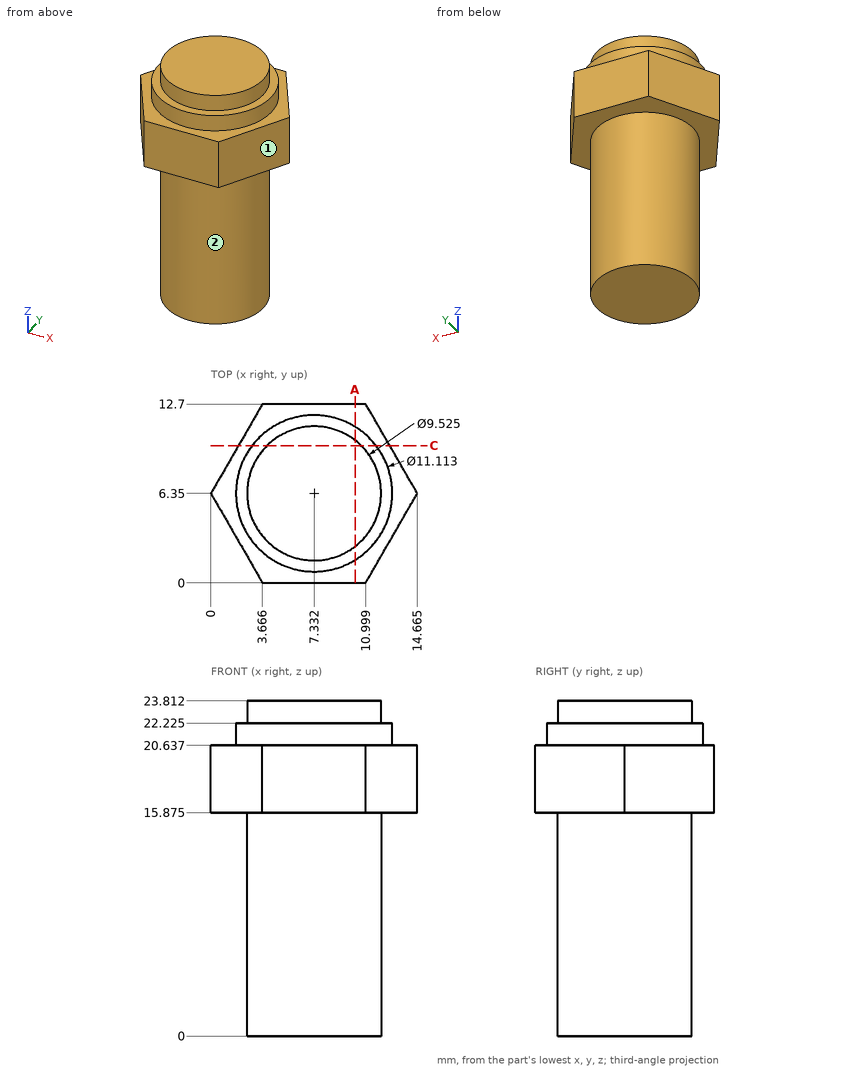
Study the drawing (mm; zero at the part's minimum x, y, z) and answer. A direction names the side the tool comes from. Coordinates: 2 decimals unless noted, no trailing zeros. Loops run counter-clockwise (first coordinate to the right, second up) from the corner with the lowest first, then second, coordinate; pieces in that order, holes last. Notation, with made-up numbers: (26.5, 68.5) -> (69.5, 68.5) arc R28 ccw to (69.5, 92.5) -> close; hole circle Ø2 at (23, 42). An arc over 180 degrees is marked (long way). Answer in a Markdown table with one row per item. Add a question column.
1. The part is cut by section C-C, the plane y = 9.75. Write down the section's boundary in (x, z) (1 decimal).
2. Flat-ended cylindrical pins translate along their axes: P1, Ø3, axis at y = 6.5, z = 18.5, coming from the +X side (1 decimal); P2, Ø3, axis at y = 3.5, z = 9.5, coming from the +X side; P3, Ø1, axis at x = 11, z = 7.5, coming from the +Y side (1 decimal). Find the tip coordinate at first contact, or state that the pin passes through.
3. For the marked faces 1 and 2, determine the directions among +Z, -Z, +X, -X, +Y, -Y from which every point of the face is accessible in a straight line to the end or side of a thin tool.
4. The part is cut by section A-A, the plane x = 10.25. Write down the section's boundary in (y, z) (1 decimal), then the cut area to 3 significant figures.
5. Consider line 1 (Z direction, x = 10.5, y = 0.5) (1 decimal); line 2 (X direction, y = 6.5, z = 4.75); line 3 (Y direction, x = 6, z = 20.75) (1 decimal). Determine where each line is inside the solid, lowest interval first. Write a range as [from, to].
Answer below:
| question | item | result |
|---|---|---|
| 1 | outline | (2, 15.9) -> (4, 15.9) -> (4, 0) -> (10.7, 0) -> (10.7, 15.9) -> (12.7, 15.9) -> (12.7, 20.6) -> (11.7, 20.6) -> (11.7, 22.2) -> (10.7, 22.2) -> (10.7, 23.8) -> (4, 23.8) -> (4, 22.2) -> (2.9, 22.2) -> (2.9, 20.6) -> (2, 20.6) -> close |
| 2 | P1 | x = 14.7 |
| 2 | P2 | x = 11.9 |
| 2 | P3 | y = 9.9 |
| 3 | face 1 | +Z, -Z, +X, -Y |
| 3 | face 2 | -Z |
| 4 | outline | (0, 15.9) -> (2.6, 15.9) -> (2.6, 0) -> (10.1, 0) -> (10.1, 15.9) -> (12.7, 15.9) -> (12.7, 20.6) -> (11.1, 20.6) -> (11.1, 22.2) -> (10.1, 22.2) -> (10.1, 23.8) -> (2.6, 23.8) -> (2.6, 22.2) -> (1.6, 22.2) -> (1.6, 20.6) -> (0, 20.6) -> close |
| 4 | area | 207 mm2 |
| 5 | line 1 | [15.9, 20.6] |
| 5 | line 2 | [2.57, 12.09] |
| 5 | line 3 | [1, 11.7] |
